from build123d import *

# Parameters (mm, degrees)
F0_W       = 137.4987065792
F0_H       = 91.6657298803
F1_DEPTH   = 76.2
F3_R       = 34.4698963813
F4_DEPTH   = 76.2
F5_R       = 33.2776122009
F1_FACE1_W = 137.4987065792
F1_FACE1_H = 91.6657298803
F6_DEPTH   = 25.4
F7_R       = 29.7028077698
F8_DEPTH   = 25.4
F9_R       = 24.8229893925
F10_DEPTH  = 25.4
F11_R      = 22.2267461951
F12_DEPTH  = 127
F13_R      = 13.2555629358
F14_DEPTH  = 127
F15_R      = 12.3283716693
F16_DEPTH  = 127
F17_R      = 13.7331139198
F19_DEPTH  = 127
F21_R      = 15.0922963459
F22_DEPTH  = 127
F23_R      = 12.709116002
F24_DEPTH  = 152.4


# Not quite as in the source:
# - a feature of the source that left no trace in its solid (it failed there, or was rolled back) is left out


with BuildPart() as f1:
    # F0 (on Front) → F1 (new body)
    with BuildSketch(Plane.XZ):
        Rectangle(F0_W, F0_H)
    extrude(amount=F1_DEPTH)

    # F3 (on Front) → F4 (cut)
    with BuildSketch(Plane.XZ):
        with Locations((0, 31.9152921438)):
            Circle(F3_R)
    extrude(amount=-F4_DEPTH, mode=Mode.SUBTRACT)

    # F5 (on Front) + F1_face1 (on face) → F6 (cut)
    with BuildSketch(Plane.XZ):
        with Locations((0, 32.8243151307)):
            Circle(F5_R)
    with BuildSketch(Plane.XZ.offset(76.2)):
        Rectangle(F1_FACE1_W, F1_FACE1_H)
    extrude(amount=-F6_DEPTH, mode=Mode.SUBTRACT)

    # F7 (on Front) → F8 (cut)
    with BuildSketch(Plane.XZ):
        with Locations((0, 34.5415323973)):
            Circle(F7_R)
    extrude(amount=-F8_DEPTH, mode=Mode.SUBTRACT)

    # F9 (on Front) → F10 (cut)
    with BuildSketch(Plane.XZ):
        with Locations((0, 21.1320593953)):
            Circle(F9_R)
    extrude(amount=-F10_DEPTH, mode=Mode.SUBTRACT)

    # F11 (on face) → F12 (cut)
    with BuildSketch(Plane.XY.offset(45.8328649402)):
        with Locations((4.9597388133, -41.3516201079)):
            Circle(F11_R)
    extrude(amount=-F12_DEPTH, mode=Mode.SUBTRACT)

    # F13 (on face) → F14 (cut)
    with BuildSketch(Plane.XZ.offset(50.8)):
        with Locations((-42.5670817494, 0)):
            Circle(F13_R)
    extrude(amount=-F14_DEPTH, mode=Mode.SUBTRACT)

    # F15 (on Front) → F16 (cut)
    with BuildSketch(Plane.XZ):
        with Locations((51.0331951082, 0)):
            Circle(F15_R)
    extrude(amount=-F16_DEPTH, mode=Mode.SUBTRACT)

    # F17 (on Front) → F19 (cut)
    with BuildSketch(Plane.XZ):
        with Locations((48.1030344963, 0)):
            Circle(F17_R)
    extrude(amount=-F19_DEPTH, mode=Mode.SUBTRACT)

    # F21 (on Front) → F22 (cut)
    with BuildSketch(Plane.XZ):
        with Locations((40.081076324, 0)):
            Circle(F21_R)
    extrude(amount=-F22_DEPTH, mode=Mode.SUBTRACT)

    # F23 (on Front) → F24 (cut)
    with BuildSketch(Plane.XZ):
        with Locations((41.4244011045, 6.4881131984)):
            Circle(F23_R)
    extrude(amount=F24_DEPTH, mode=Mode.SUBTRACT)


solid = f1.part
Can you work these out from the model? Positions are in its coordinate system, mm. Give positions to 0.01 mm unless a question says otherwise; leave off trailing zeros. Loops run counter-clockwise (first coordinate to the right, second up) from the corner with the lowest first, then second, coordinate; pieces in that order, holes last. Notation, with made-up numbers: M -34,-38 L 22,-38 A19 ccw 22,-20 Z; hole C 80.25,0.5 d4. An arc over 180 degrees is marked long. One line per item, written item: value.
1) Imagine slicing it at D-D on z = -32. Write out the boundary of the cut face in (x, y), and give its area (3 significant figures).
Geometry check:
outline: M -68.75,-50.8 L -15.16,-50.8 A22.23 cw long 25.08,-50.8 L 68.75,-50.8 L 68.75,0 L -68.75,0 Z
area: 5,800 mm²
2) Imagine slicing it at B-B on z = 0. Write out the boundary of the cut face in (x, y), and give its area (3 significant figures).
Geometry check:
outline: M -68.75,-50.8 L -55.82,-50.8 L -55.82,0 L -68.75,0 Z; M -29.31,-50.8 L -15.16,-50.8 A22.23 cw long 25.08,-50.8 L 30.5,-50.8 L 30.5,0 L -29.31,0 Z; M 52.35,-50.8 L 68.75,-50.8 L 68.75,0 L 52.35,0 Z
area: 3,340 mm²
3) Thinking about a two-plate mould opening in X: for faces 1 (the face through (53.547, -25.044, 10.306)), 2 (the face through (68.749, -25, -1)), 3 (the face through (5.585, -19.134, 0.642)), 4 (the face through (-1, 0, 1)), which applies, +X half, -X half, draft (parallel to the pull), parting line (faces both ways), or undercut?
Geometry check:
face 1: undercut
face 2: +X half
face 3: undercut
face 4: draft
4) Please list where these lines run through material, in increasing order: line 1 (X direction, y = -22, z = 14.5); line 2 (X direction, y = -14, z = 11.5); line 3 (X direction, y = -31.5, z = 2.5).
Geometry check:
line 1: x = -68.75 to -5.97, 15.89 to 31.56, 51.29 to 68.75
line 2: x = -68.75 to -49.16, -35.97 to 29.75, 53.1 to 68.75
line 3: x = -68.75 to -55.58, -29.55 to -14.96, 24.88 to 29.36, 53.49 to 68.75
5) Imagine slicing it at C-C on x = -36.5. Write out the boundary of the cut face in (y, z).
Geometry check:
outline: M -50.8,-45.83 L 0,-45.83 L 0,-11.79 L -50.8,-11.79 Z; M -50.8,11.79 L 0,11.79 L 0,45.83 L -50.8,45.83 Z
6) Imagine slicing it at A-A on y = -41. Write out the boundary of the cut face in (x, z).
Geometry check:
outline: M -68.75,-45.83 L -17.26,-45.83 L -17.26,45.83 L -68.75,45.83 Z; M 27.18,-45.83 L 68.75,-45.83 L 68.75,45.83 L 27.18,45.83 Z; hole C -42.57,0 d26.51; hole C 41.42,6.49 d25.42
